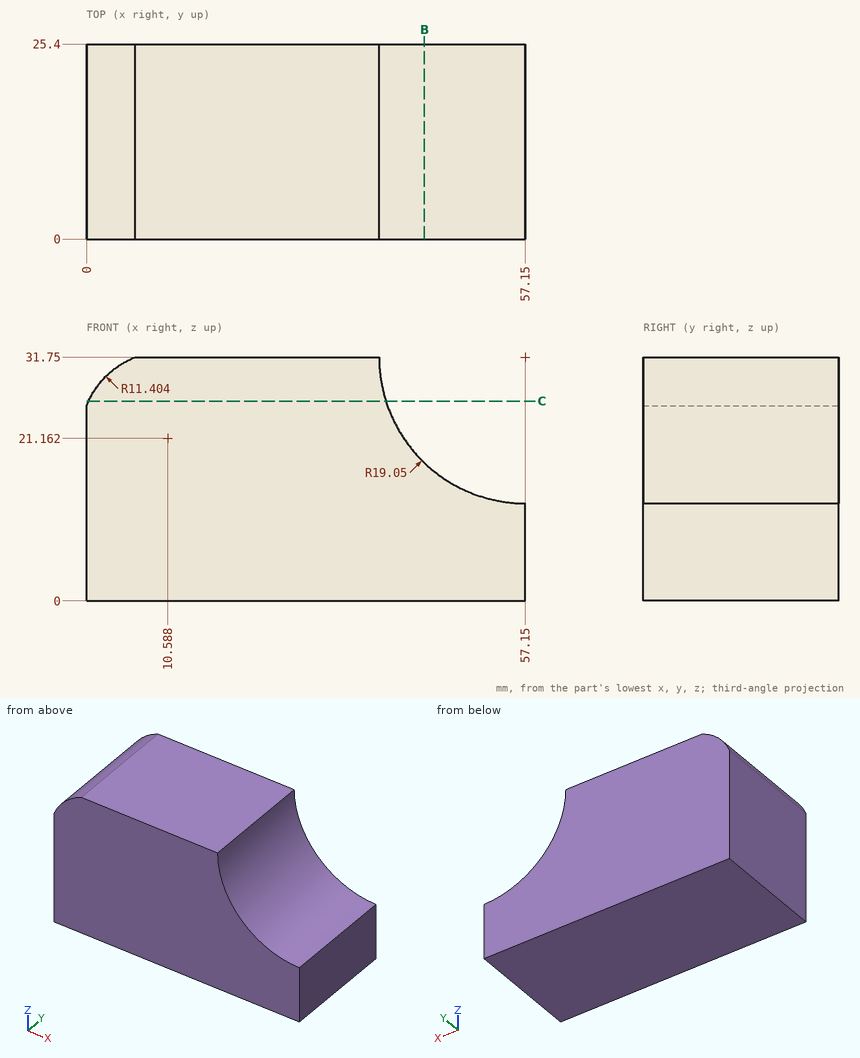
Check sheet for the drawn part. Datum: minimum x, y, z corner. Units: mm. Round coordinates to 2 decimals unless told otherwise and drop trailing zeros. Loops run counter-clockwise (first coordinate to the right, second up) from the corner with the lowest first, then second, coordinate; pieces in that order, holes last. Notation, with made-up numbers: (23.25, -17) - (29.25, -17) arc R28 cw to (29.25, 14) - close; hole circle Ø9 at (-20, -6). An arc over 180 degrees is marked (long way). Write item = value, one per line. Start each with the question number.
1. Depth check by flat-ended pin: pin 1 (6 mm diameter, centred on y = 18, z = 20, fed in from +X) (1 decimal). Enter the tip coordinate at first touch or a pass-through.
2. Section check C-C on z = 26. Enter the section's corners in (x, y).
3. Section check B-B on x = 44. Enter the section's corners in (y, z).
4. Thickness scan on line 1 (X direction, y = 17.5, z = 23); line 2 (X direction, y = 9, z = 30.5); line 3 (Z direction, x = 47, y = 18.25). Record the ranges inside material, lowest first.
Working result:
q1.pin_1 = 45.1
q2.outline = (0.26, 0) - (38.99, 0) - (38.99, 25.4) - (0.26, 25.4) - close
q3.outline = (0, 0) - (25.4, 0) - (25.4, 17.97) - (0, 17.97) - close
q4.line_1 = 0 to 40.23
q4.line_2 = 4.04 to 38.14
q4.line_3 = 0 to 15.63
